Design review of the part built by this model. Coordinates are the model's own, in mm. A direction names the side the tool comes from. Round coordinates to 2 decimals unless told otherwise and drop trailing zeros. Write each loop counter-clockwise with the first axis right and the second up, starting at its lowest first coordinate (ties: lowest second). Pieces come first, ordered by that corner, then holes. Notation, with made-up numbers: (-24.5, 38.5) -> (-18.5, 38.5) arc R23 cw to (-18.5, 64.5) -> close; hole circle Ø1 at (88, 45). An arc over 180 degrees is marked (long way). One line per question, with ' | ' between items. Start each with the question number.
1) For faces 5 (the cylindrical face through (11.54, 5.62, 1.57)), 6 (the cylindrical face through (11.328, -6.033, 1.565)), 7 (the cylindrical face through (-11.328, 6.033, 1.565)), 8 (the cylindrical face through (11.808, -7.466, 1.565)), 9 (the cylindrical face through (-0.124, -12.8, 1.565)), list the 3-axis set-ups (+Z, -Z, +X, -X, +Y, -Y) from which the entire face can be reached by the end or side of a thin tool; tool diameter is ignored.
2) For probe 1 along Y at (x, z) = (-10.5, 1.8); probe 2 along Y at (x, z) = (12.75, 0.1); probe 3 along Y at (x, z) = (-11.5, 2.5), list the stretches that pass through material, from the lowest coordinate up.
3) Consider section A-A (y = 0). Give the boundary of the cut face in (x, z) (1 decimal), then the cut area to 3 significant figures.
4) Mouldability with a two-part tool opening along Y and no side actions: class faces 1 (the cylindrical face through (-7.624, -10.283, 1.565)), 2 (the cylindrical face through (-0.9, 13.94, 1.57)), 3 (the cylindrical face through (-5.62, 11.54, 1.57)), 4 (the cylindrical face through (-9.24, -8.91, 1.57)) as +Y half, -Y half, draft (parallel to the pull), parting line (faces both ways), or undercut.
5) Insertion check: pin 1 Ø1.5 at (x, z) = (-3.5, 3) entering from +Y; pin 2 Ø1 at (x, z) = (8, 1) entering from +Y. Each pin has a flat end and moves straight along its axis. Give the tip position at first contact, or say it passes through.
```python
from build123d import *

# Parameters (mm, degrees)
SKETCH3_R         = 13.97
GEARBODY_DEPTH    = 3.175
TOOTHCUT_DEPTH    = 21.010058096
CIRPATTERN1_COUNT = 20
BOREDIA_R         = 1.460500026
BORE_DEPTH        = 12700


with BuildPart() as part:
    # Sketch3 → gearBody (new body)
    with BuildSketch(Plane.XY):
        Circle(SKETCH3_R)
    extrude(amount=GEARBODY_DEPTH)

    # Sketch2 → toothCut (cut, through all)
    with BuildSketch(Plane.XY):
        with BuildLine():
            ThreePointArc((11.055114421, -1.246803989), (11.078104947, -1.022578023), (11.09654807, -0.797932304))
            ThreePointArc((11.09654807, -0.797932304), (11.248380712, -0.471754036), (11.578721183, -0.329203743))
            ThreePointArc((11.578721183, -0.329203743), (13.810169569, 0.302046563), (15.522633304, 1.865794244))
            ThreePointArc((15.522633304, 1.865794244), (15.568180658, -1.437039952), (14.918810012, -4.675728892))
            ThreePointArc((14.918810012, -4.675728892), (13.521529943, -2.824932507), (11.443338244, -1.795875603))
            ThreePointArc((11.443338244, -1.795875603), (11.144673729, -1.595264236), (11.055114421, -1.246803989))
        make_face()
    toothcut = extrude(amount=TOOTHCUT_DEPTH, mode=Mode.SUBTRACT)

    # CirPattern1: toothCut ×20 about axis
    cirpattern1_axis = Axis((0, 0, 0), (0, 0, 1))
    for i in range(1, CIRPATTERN1_COUNT):
        add(toothcut.rotate(cirpattern1_axis, i * 360 / CIRPATTERN1_COUNT), mode=Mode.SUBTRACT)

    # boreDia → bore (cut, symmetric)
    with BuildSketch(Plane.XY):
        Circle(BOREDIA_R)
    extrude(amount=BORE_DEPTH, both=True, mode=Mode.SUBTRACT)


solid = part.part
```
From the geometry:
1) face 5: +Z, -Z | face 6: +Z, -Z, +X | face 7: +Z, -Z, -X | face 8: +Z, -Z, +X, -Y | face 9: +Z, -Z, -Y
2) probe 1: y = -9.21 to -7.52, -5.35 to 3.95, 5.35 to 7.69 | probe 2: y = -4.05 to -2.3, -0.14 to 1.77, 4.27 to 5.65 | probe 3: y = -5.61 to -3.43, -1.83 to 0.34, 1.81 to 4.02, 6.22 to 7.89
3) outline: (-13.2, 0) -> (-1.5, 0) -> (-1.5, 3.2) -> (-13.2, 3.2) -> close; (1.5, 0) -> (13.2, 0) -> (13.2, 3.2) -> (1.5, 3.2) -> close | area: 74.3 mm2
4) face 1: undercut | face 2: +Y half | face 3: undercut | face 4: -Y half
5) pin 1: stops at y = 12.73 | pin 2: stops at y = 11.79
